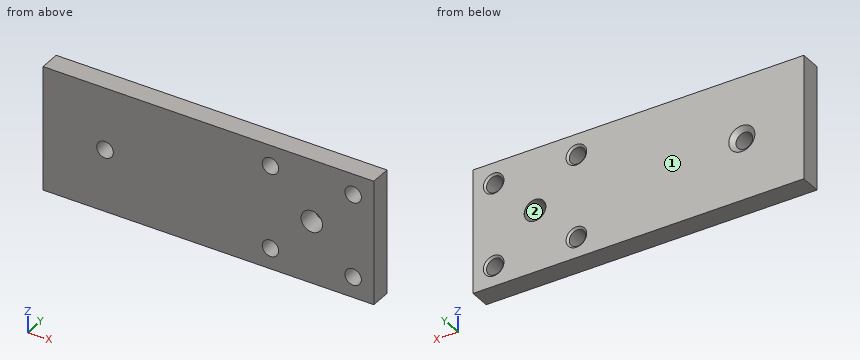
```python
from build123d import *

# Parameters (mm, degrees)
SKETCH1_W                            = 101.6
SKETCH1_H                            = 38.1
BOSS_EXTRUDE1_DEPTH                  = 6.35
F_1_4_20_TAPPED_HOLE1_D              = 5.1054
F_1_4_20_TAPPED_HOLE1_CSINK_D        = 8.0264
F_1_4_20_TAPPED_HOLE1_CSINK_ANGLE    = 100
M6_CLEARANCE_HOLE1_D                 = 6.6
M6_CLEARANCE_HOLE1_CSINK_D           = 6.65
M6_CLEARANCE_HOLE1_CSINK_ANGLE       = 100
F_8_0_199_DIAMETER_HOLE1_D           = 5.0546
F_8_0_199_DIAMETER_HOLE1_CSINK_D     = 6.3246
F_8_0_199_DIAMETER_HOLE1_CSINK_ANGLE = 100


with BuildPart() as part:
    # Sketch1 → Boss-Extrude1 (new body)
    with BuildSketch(Plane(origin=(0, 0, 0), x_dir=(1, 0, 0), z_dir=(0, 1, 0))):
        with Locations((50.8, 19.05)):
            Rectangle(SKETCH1_W, SKETCH1_H)
    extrude(amount=BOSS_EXTRUDE1_DEPTH)

    # 1/4-20 Tapped Hole1 (through all)
    with Locations(Plane(origin=(0, 6.35, 0), x_dir=(1, 0, 0), z_dir=(0, 1, 0))):
        with Locations((19.05, 19.05)):
            CounterSinkHole(F_1_4_20_TAPPED_HOLE1_D / 2, F_1_4_20_TAPPED_HOLE1_CSINK_D / 2, counter_sink_angle=F_1_4_20_TAPPED_HOLE1_CSINK_ANGLE)

    # M6 Clearance Hole1 (through all)
    with Locations(Plane(origin=(0, 6.35, 0), x_dir=(1, 0, 0), z_dir=(0, 1, 0))):
        with Locations((82.55, 19.05)):
            CounterSinkHole(M6_CLEARANCE_HOLE1_D / 2, M6_CLEARANCE_HOLE1_CSINK_D / 2, counter_sink_angle=M6_CLEARANCE_HOLE1_CSINK_ANGLE)

    # #8 (0.199) Diameter Hole1 (through all)
    with Locations(Plane(origin=(0, 6.35, 0), x_dir=(1, 0, 0), z_dir=(0, 1, 0))):
        with Locations((95.25, 31.75), (69.85, 31.75), (69.85, 6.35), (95.25, 6.35)):
            CounterSinkHole(F_8_0_199_DIAMETER_HOLE1_D / 2, F_8_0_199_DIAMETER_HOLE1_CSINK_D / 2, counter_sink_angle=F_8_0_199_DIAMETER_HOLE1_CSINK_ANGLE)


solid = part.part
```
The model under review builds one solid part; all positions refer to its coordinate system, in mm. Face numbers are marked on the shaded views. Round coordinates to 2 decimals unless told otherwise and drop trailing zeros. Write each loop counter-clockwise with the first axis right and the second up, starting at its lowest first coordinate (ties: lowest second). Pieces come first, ordered by that corner, then holes. Notation, with made-up numbers: (52, 65.25) - (98, 65.25) arc R29 cw to (98, 85.25) - close; hole circle Ø5 at (10, -19.75). An arc over 180 degrees is marked (long way). Answer as CSV lines item,"result". Start each with the question number.
(1) Draft analysis for pull direction X (two halves, no side actions). For the marked faces 1 and 2, state which applies: pulls with the +X half, pulls with the -X half, needs draft (parallel to the pull), parting line crosses it, or undercut.
(2) We need section C-C on x = 82.55. State the section outline as (y, z) points (3 decimals).
(3) We need section B-B on y = 3.75. State the section outline as (x, z) points, plus the area to 3 significant figures.
(4) To check wall thickness, follow line 1 (Z direction, x = 69.85, y = 2.2); line 2 (X direction, y = 1.65, z = -31.75); line 3 (Z direction, x = 19.05, y = 1.6). State the ranges of each line that lie inside material, in increasing order.
(5) We need section D-D on x = 95.25. State the section outline as (y, z) points, plus the area to 3 significant figures.
(6) We need section A-A on z = -19.05. Give the number of separate pieces and of enclosed holes in the cut face, plus the area to 3 significant figures.
(7) For pin 1 Ø6 at (x, z) = (69.85, -6.35) entering from +Y; pin 2 Ø8 at (x, z) = (95.25, -31.75) entering from +Y; pin 3 Ø6.5 at (x, z) = (19.05, -19.05) entering from +Y, all flat-tipped, find the tip position at first contact; note any pin that passes through.
Worked answers:
1,face 1,"needs draft"
1,face 2,"undercut"
2,outline,"(0, -38.1) - (6.35, -38.1) - (6.35, -22.375) - (6.329, -22.35) - (0, -22.35) - close; (0, -15.75) - (6.329, -15.75) - (6.35, -15.725) - (6.35, 0) - (0, 0) - close"
3,outline,"(0, -38.1) - (101.6, -38.1) - (101.6, 0) - (0, 0) - close; hole circle Ø5.11 at (19.05, -19.05); hole circle Ø5.05 at (69.85, -31.75); hole circle Ø5.05 at (69.85, -6.35); hole circle Ø6.6 at (82.55, -19.05); hole circle Ø5.05 at (95.25, -31.75); hole circle Ø5.05 at (95.25, -6.35)"
3,area,"3,740 mm²"
4,line 1,"-38.1 to -34.28, -29.22 to -8.88, -3.82 to 0"
4,line 2,"0 to 67.32, 72.38 to 92.72, 97.78 to 101.6"
4,line 3,"-38.1 to -21.6, -16.5 to 0"
5,outline,"(0, -38.1) - (6.35, -38.1) - (6.35, -34.91) - (5.82, -34.28) - (0, -34.28) - close; (0, -29.22) - (5.82, -29.22) - (6.35, -28.59) - (6.35, -9.51) - (5.82, -8.88) - (0, -8.88) - close; (0, -3.82) - (5.82, -3.82) - (6.35, -3.19) - (6.35, 0) - (0, 0) - close"
5,area,"177 mm²"
6,separate pieces,"3"
6,enclosed holes,"0"
6,area,"569 mm²"
7,pin 1,"y = 6.21"
7,pin 2,"y = 6.35"
7,pin 3,"y = 5.71"
